Here's how the part is built. I have some questions about the finished solid (model axes, mm). Coordinates: 2 decimals unless noted, no trailing zeros. Loops run counter-clockwise (first coordinate to the right, second up) from the corner with the lowest first, then second, coordinate; pieces in that order, holes last.
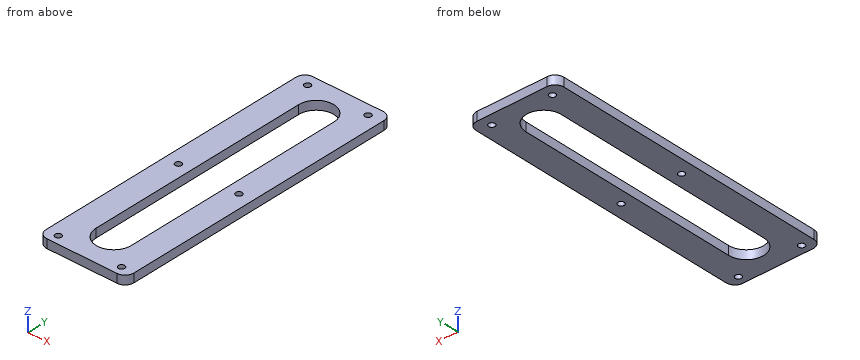
from build123d import *

# Parameters (mm, degrees)
SKETCH1_W             = 31.75
SKETCH1_H             = 106.68
BOSS_EXTRUDE1_DEPTH   = 3.175
FILLET1_R             = 3.175
F_4_40_TAPPED_HOLE1_D = 2.2606


with BuildPart() as part:
    # Sketch1 → Boss-Extrude1 (new body)
    with BuildSketch(Plane.XY.offset(3.175)):
        with Locations((15.875, 53.34)):
            Rectangle(SKETCH1_W, SKETCH1_H)
        with BuildLine():
            Line((22.225, 93.98), (22.225, 12.7))
            ThreePointArc((22.225, 12.7), (15.875, 6.35), (9.525, 12.7))
            Line((9.525, 12.7), (9.525, 93.98))
            ThreePointArc((9.525, 93.98), (15.875, 100.33), (22.225, 93.98))
        make_face(mode=Mode.SUBTRACT)
    extrude(amount=-BOSS_EXTRUDE1_DEPTH)

    # Fillet1
    fillet1_edges = [part.edges().sort_by_distance(p)[0] for p in [
        (0, 0, 1.5875),
        (0, 106.68, 1.5875),
        (31.75, 106.68, 1.5875),
        (31.75, 0, 1.5875),
    ]]
    fillet(fillet1_edges, radius=FILLET1_R)

    # #4-40 Tapped Hole1 (through all)
    with Locations(Plane(origin=(0, 0, 0), x_dir=(-1, 0, 0), z_dir=(0, 0, -1))):
        with Locations((-4.445, 3.175), (-4.9403, 50.8), (-27.305, 3.175), (-26.8097, 50.8), (-26.8097, 102.616), (-4.9403, 102.616)):
            Hole(F_4_40_TAPPED_HOLE1_D / 2)


solid = part.part
Q1. Suppose I cut it at D-D on z = 0.85. Write out the boundary of the cut face in (x, y) (3 decimals).
Q2. Please list where these lines run through material, in increasing order: probe 1 along X at (y, z) = (71, 2.75) (3 decimals); probe 2 along X at (y, z) = (51.5, 0.7) (3 decimals); probe 3 along Y at (x, z) = (15.5, 2.3).
Q3. Suppose I cut it at A-A on y = 77. Write out the boundary of the cut face in (x, z) (3 decimals).
Q4. Suppose I cut it at B-B on x = 15.5. Write out the boundary of the cut face in (y, z) (3 decimals).
Q5. Will this pin go through, and if not, where does the flat tip stop? P1, Ø6, axis at x = 14, y = 48, coming from the +Z side.
Q6. Suppose I cut it at C-C on y = 50.8. Write out the boundary of the cut face in (x, z) (3 decimals).
Check values:
1. outline: (0, 3.175) arc R3.175 ccw to (3.175, 0) - (28.575, 0) arc R3.175 ccw to (31.75, 3.175) - (31.75, 103.505) arc R3.175 ccw to (28.575, 106.68) - (3.175, 106.68) arc R3.175 ccw to (0, 103.505) - close; hole circle Ø2.261 at (4.445, 3.175); hole circle Ø2.261 at (4.94, 50.8); hole circle Ø2.261 at (4.94, 102.616); hole (9.525, 12.7) arc R6.35 ccw to (22.225, 12.7) - (22.225, 93.98) arc R6.35 ccw to (9.525, 93.98) - close; hole circle Ø2.261 at (26.81, 50.8); hole circle Ø2.261 at (26.81, 102.616); hole circle Ø2.261 at (27.305, 3.175)
2. probe 1: x = 0 to 9.525, 22.225 to 31.75
2. probe 2: x = 0 to 4.053, 5.828 to 9.525, 22.225 to 25.922, 27.697 to 31.75
2. probe 3: y = 0 to 6.36, 100.32 to 106.68
3. outline: (0, 0) - (9.525, 0) - (9.525, 3.175) - (0, 3.175) - close; (22.225, 0) - (31.75, 0) - (31.75, 3.175) - (22.225, 3.175) - close
4. outline: (0, 0) - (6.361, 0) - (6.361, 3.175) - (0, 3.175) - close; (100.319, 0) - (106.68, 0) - (106.68, 3.175) - (100.319, 3.175) - close
5. P1: passes through
6. outline: (0, 0) - (3.81, 0) - (3.81, 3.175) - (0, 3.175) - close; (6.071, 0) - (9.525, 0) - (9.525, 3.175) - (6.071, 3.175) - close; (22.225, 0) - (25.679, 0) - (25.679, 3.175) - (22.225, 3.175) - close; (27.94, 0) - (31.75, 0) - (31.75, 3.175) - (27.94, 3.175) - close
